Could you check a few things on this model? Use its own coordinates, in mm. A direction names the side the tool comes from. Round coordinates to 2 decimals unless told otherwise and drop trailing zeros. Loops run counter-clockwise (first coordinate to the right, second up) from the corner with the lowest first, then second, coordinate; pieces in that order, holes last.
from build123d import *

# Parameters (mm, degrees)
BOSS_EXTRUDE1_DEPTH = 30
SKETCH2_R           = 11.5
BOSS_EXTRUDE2_DEPTH = 3
CUT_EXTRUDE1_DEPTH  = 37.789944278


with BuildPart() as part:
    # Sketch1 → Boss-Extrude1 (new body)
    with BuildSketch(Plane(origin=(0, 0, 0), x_dir=(1, 0, 0), z_dir=(0, 1, 0))):
        with BuildLine():
            Line((-4, -1), (-4, 1))
            ThreePointArc((-4, 1), (0, 5), (4, 1))
            Line((4, 1), (4, -1))
            ThreePointArc((4, -1), (0, -5), (-4, -1))
        make_face()
        with BuildLine():
            Line((-2, -0.8), (-2, 0.8))
            ThreePointArc((-2, 0.8), (0, 2.8), (2, 0.8))
            Line((2, 0.8), (2, -0.8))
            ThreePointArc((2, -0.8), (0, -2.8), (-2, -0.8))
        make_face(mode=Mode.SUBTRACT)
    extrude(amount=BOSS_EXTRUDE1_DEPTH)

    # Sketch2 → Boss-Extrude2 (add)
    with BuildSketch(Plane(origin=(0, 30, 0), x_dir=(1, 0, 0), z_dir=(0, 1, 0))):
        with Locations(Location((0, 0, 0), (0, 0, 270))):
            Circle(SKETCH2_R)
    extrude(amount=BOSS_EXTRUDE2_DEPTH)

    # Sketch3 → Cut-Extrude1 (cut, through all)
    with BuildSketch(Plane(origin=(0, 33, 0), x_dir=(1, 0, 0), z_dir=(0, 1, 0))):
        with BuildLine():
            Line((-1, 10.5), (-1, 17.5))
            ThreePointArc((-1, 17.5), (0, 18.5), (1, 17.5))
            Line((1, 17.5), (1, 10.5))
            ThreePointArc((1, 10.5), (0, 9.5), (-1, 10.5))
        make_face()
        with BuildLine():
            Line((2.651518884, 10.208792662), (5.045659887, 16.786641007))
            ThreePointArc((5.045659887, 16.786641007), (6.327372652, 17.384313485), (6.925045129, 16.10260072))
            Line((6.925045129, 16.10260072), (4.530904126, 9.524752375))
            ThreePointArc((4.530904126, 9.524752375), (3.249191362, 8.927079897), (2.651518884, 10.208792662))
        make_face()
        with BuildLine():
            Line((5.983225459, 8.686254262), (10.482738726, 14.048565364))
            ThreePointArc((10.482738726, 14.048565364), (11.891570779, 14.171822198), (12.014827613, 12.762990145))
            Line((12.014827613, 12.762990145), (7.515314345, 7.400679043))
            ThreePointArc((7.515314345, 7.400679043), (6.106482292, 7.27742221), (5.983225459, 8.686254262))
        make_face()
        with BuildLine():
            Line((8.59326674, 6.116025404), (14.655444566, 9.616025404))
            ThreePointArc((14.655444566, 9.616025404), (16.02146997, 9.25), (15.655444566, 7.883974596))
            Line((15.655444566, 7.883974596), (9.59326674, 4.383974596))
            ThreePointArc((9.59326674, 4.383974596), (8.227241336, 4.75), (8.59326674, 6.116025404))
        make_face()
        with BuildLine():
            Line((10.166833229, 2.808113619), (17.0604875, 4.023650862))
            ThreePointArc((17.0604875, 4.023650862), (18.218943431, 3.212491287), (17.407783855, 2.054035356))
            Line((17.407783855, 2.054035356), (10.514129584, 0.838498112))
            ThreePointArc((10.514129584, 0.838498112), (9.355673654, 1.649657688), (10.166833229, 2.808113619))
        make_face()
        with BuildLine():
            Line((10.514129584, -0.838498112), (17.407783855, -2.054035356))
            ThreePointArc((17.407783855, -2.054035356), (18.218943431, -3.212491287), (17.0604875, -4.023650862))
            Line((17.0604875, -4.023650862), (10.166833229, -2.808113619))
            ThreePointArc((10.166833229, -2.808113619), (9.355673654, -1.649657688), (10.514129584, -0.838498112))
        make_face()
        with BuildLine():
            Line((9.59326674, -4.383974596), (15.655444566, -7.883974596))
            ThreePointArc((15.655444566, -7.883974596), (16.02146997, -9.25), (14.655444566, -9.616025404))
            Line((14.655444566, -9.616025404), (8.59326674, -6.116025404))
            ThreePointArc((8.59326674, -6.116025404), (8.227241336, -4.75), (9.59326674, -4.383974596))
        make_face()
        with BuildLine():
            Line((7.515314345, -7.400679043), (12.014827613, -12.762990145))
            ThreePointArc((12.014827613, -12.762990145), (11.891570779, -14.171822198), (10.482738726, -14.048565364))
            Line((10.482738726, -14.048565364), (5.983225459, -8.686254262))
            ThreePointArc((5.983225459, -8.686254262), (6.106482292, -7.27742221), (7.515314345, -7.400679043))
        make_face()
        with BuildLine():
            Line((4.530904126, -9.524752375), (6.925045129, -16.10260072))
            ThreePointArc((6.925045129, -16.10260072), (6.327372652, -17.384313485), (5.045659887, -16.786641007))
            Line((5.045659887, -16.786641007), (2.651518884, -10.208792662))
            ThreePointArc((2.651518884, -10.208792662), (3.249191362, -8.927079897), (4.530904126, -9.524752375))
        make_face()
        with BuildLine():
            Line((1, -10.5), (1, -17.5))
            ThreePointArc((1, -17.5), (0, -18.5), (-1, -17.5))
            Line((-1, -17.5), (-1, -10.5))
            ThreePointArc((-1, -10.5), (0, -9.5), (1, -10.5))
        make_face()
        with BuildLine():
            Line((-2.651518884, -10.208792662), (-5.045659887, -16.786641007))
            ThreePointArc((-5.045659887, -16.786641007), (-6.327372652, -17.384313485), (-6.925045129, -16.10260072))
            Line((-6.925045129, -16.10260072), (-4.530904126, -9.524752375))
            ThreePointArc((-4.530904126, -9.524752375), (-3.249191362, -8.927079897), (-2.651518884, -10.208792662))
        make_face()
        with BuildLine():
            Line((-5.983225459, -8.686254262), (-10.482738726, -14.048565364))
            ThreePointArc((-10.482738726, -14.048565364), (-11.891570779, -14.171822198), (-12.014827613, -12.762990145))
            Line((-12.014827613, -12.762990145), (-7.515314345, -7.400679043))
            ThreePointArc((-7.515314345, -7.400679043), (-6.106482292, -7.27742221), (-5.983225459, -8.686254262))
        make_face()
        with BuildLine():
            Line((-8.59326674, -6.116025404), (-14.655444566, -9.616025404))
            ThreePointArc((-14.655444566, -9.616025404), (-16.02146997, -9.25), (-15.655444566, -7.883974596))
            Line((-15.655444566, -7.883974596), (-9.59326674, -4.383974596))
            ThreePointArc((-9.59326674, -4.383974596), (-8.227241336, -4.75), (-8.59326674, -6.116025404))
        make_face()
        with BuildLine():
            Line((-10.166833229, -2.808113619), (-17.0604875, -4.023650862))
            ThreePointArc((-17.0604875, -4.023650862), (-18.218943431, -3.212491287), (-17.407783855, -2.054035356))
            Line((-17.407783855, -2.054035356), (-10.514129584, -0.838498112))
            ThreePointArc((-10.514129584, -0.838498112), (-9.355673654, -1.649657688), (-10.166833229, -2.808113619))
        make_face()
        with BuildLine():
            Line((-10.514129584, 0.838498112), (-17.407783855, 2.054035356))
            ThreePointArc((-17.407783855, 2.054035356), (-18.218943431, 3.212491287), (-17.0604875, 4.023650862))
            Line((-17.0604875, 4.023650862), (-10.166833229, 2.808113619))
            ThreePointArc((-10.166833229, 2.808113619), (-9.355673654, 1.649657688), (-10.514129584, 0.838498112))
        make_face()
        with BuildLine():
            Line((-9.59326674, 4.383974596), (-15.655444566, 7.883974596))
            ThreePointArc((-15.655444566, 7.883974596), (-16.02146997, 9.25), (-14.655444566, 9.616025404))
            Line((-14.655444566, 9.616025404), (-8.59326674, 6.116025404))
            ThreePointArc((-8.59326674, 6.116025404), (-8.227241336, 4.75), (-9.59326674, 4.383974596))
        make_face()
        with BuildLine():
            Line((-7.515314345, 7.400679043), (-12.014827613, 12.762990145))
            ThreePointArc((-12.014827613, 12.762990145), (-11.891570779, 14.171822198), (-10.482738726, 14.048565364))
            Line((-10.482738726, 14.048565364), (-5.983225459, 8.686254262))
            ThreePointArc((-5.983225459, 8.686254262), (-6.106482292, 7.27742221), (-7.515314345, 7.400679043))
        make_face()
        with BuildLine():
            Line((-4.530904126, 9.524752375), (-6.925045129, 16.10260072))
            ThreePointArc((-6.925045129, 16.10260072), (-6.327372652, 17.384313485), (-5.045659887, 16.786641007))
            Line((-5.045659887, 16.786641007), (-2.651518884, 10.208792662))
            ThreePointArc((-2.651518884, 10.208792662), (-3.249191362, 8.927079897), (-4.530904126, 9.524752375))
        make_face()
    extrude(amount=-CUT_EXTRUDE1_DEPTH, mode=Mode.SUBTRACT)


solid = part.part
Item 1: If we section it at A-A, the plane y = 23: Please give me the cut outline in (x, z), then the cut area to 3 significant figures.
Results list:
outline: (-4, -1) arc R4 ccw to (4, -1) - (4, 1) arc R4 ccw to (-4, 1) - close; hole (-2, -0.8) arc R2 ccw to (2, -0.8) - (2, 0.8) arc R2 ccw to (-2, 0.8) - close
area: 47.3 mm2
Item 2: Will these pins go through, and if not, where does the flat tip stop? pin 1 (4 mm diameter, centred on x = 1.5, y = 11.5, fed in from -Z); pin 2 (0.5 mm diameter, centred on y = 31.5, z = 11, fed in from -X); pin 3 (5 mm diameter, centred on y = 11.5, z = -3.5, fed in from +X).
Results list:
pin 1: stops at z = -5
pin 2: stops at x = -2.98
pin 3: stops at x = 4
Item 3: If I drill on line 1 along X through (y, z) = (7, -0.5); line 2 along Y through (x, z) = (-7, 2.75); line 3 along Z through (x, y) = (1.75, 18.5), over which ranges is the centre line in solid material (lowest first)?
Results list:
line 1: x = -4 to -2, 2 to 4
line 2: y = 30 to 33
line 3: z = -4.6 to -1.77, 1.77 to 4.6
Item 4: If we section it at B-B, the plane x = 0: Please give me the cut outline in (y, z).
Results list:
outline: (0, -5) - (30, -5) - (30, -9.5) - (33, -9.5) - (33, 9.5) - (30, 9.5) - (30, 5) - (0, 5) - (0, 2.8) - (30, 2.8) - (30, -2.8) - (0, -2.8) - close
Item 5: We'd pull the mould along Z, two halves only. Please class faces 6 (the cylindrical face through (-2.011, 31.479, 11.323)), 7 (the cylindrical face through (0, 14.8, 2.8)), 8 (the flat face through (-5, 30, 0)), 9 (the cylindrical face through (-1.98, 31.48, -11.33)): released by +Z, released by -Z, zero draft, split by the parting line, or undercut.
Results list:
face 6: released by +Z
face 7: undercut
face 8: zero draft
face 9: released by -Z
Item 6: For faces 1 (the flat face through (-10.992, 31.521, 0.923)), 2 (the flat face through (3, 0, 0)), 3 (the flat face through (-1, 32, -11)), 4 (the flat face through (-10.013, 31.521, 4.626)), 5 (the cylindrical face through (-11.5, 31.5, 0)), which set-ups out of +Z, -Z, +X, -X, +Y, -Y let a thin tool reach every point of the face, with its end or its side?
Results list:
face 1: +Y, -Y
face 2: +Z, -Z, +X, -X, -Y
face 3: -Z, +Y, -Y
face 4: +Z, +Y, -Y
face 5: -X, +Y, -Y
